from build123d import *

# Parameters (mm, degrees)
SKETCH_1_R      = 15
SKETCH_1_R_2    = 2.1
EXTRUDE_1_DEPTH = 7
EXTRUDE_START   = -2
SKETCH_2_R      = 17.5
SKETCH_2_R_2    = 2.1
EXTRUDE_2_DEPTH = 2
SKETCH_5_R      = 17.5
SKETCH_5_R_2    = 2.1
EXTRUDE_4_DEPTH = 1


with BuildPart() as part:
    # 草图1 → 凸台-拉伸1 (new body)
    with BuildSketch(Plane.XY):
        Circle(SKETCH_1_R)
        with Locations((0, 12)):
            Circle(SKETCH_1_R_2, mode=Mode.SUBTRACT)
        with Locations((10.392304845, 6)):
            Circle(SKETCH_1_R_2, mode=Mode.SUBTRACT)
        with Locations((10.392304845, -6)):
            Circle(SKETCH_1_R_2, mode=Mode.SUBTRACT)
        with Locations((0, -12)):
            Circle(SKETCH_1_R_2, mode=Mode.SUBTRACT)
        with Locations((-10.392304845, -6)):
            Circle(SKETCH_1_R_2, mode=Mode.SUBTRACT)
        with Locations((-10.392304845, 6)):
            Circle(SKETCH_1_R_2, mode=Mode.SUBTRACT)
        with Locations((4.425, 7.664324823)):
            Circle(SKETCH_1_R_2, mode=Mode.SUBTRACT)
        with Locations((4.419693866, -7.655134331)):
            Circle(SKETCH_1_R_2, mode=Mode.SUBTRACT)
        with Locations((-8.844693866, 0.009190493)):
            Circle(SKETCH_1_R_2, mode=Mode.SUBTRACT)
    extrude(amount=EXTRUDE_1_DEPTH)

    # 草图2 → 凸台-拉伸2 (add)
    with BuildSketch(Plane.XY.offset(7).offset(EXTRUDE_START)):
        Circle(SKETCH_2_R)
        with Locations((-8.844693866, 0.009190493)):
            Circle(SKETCH_2_R_2, mode=Mode.SUBTRACT)
        with Locations((-10.392304845, -6)):
            Circle(SKETCH_2_R_2, mode=Mode.SUBTRACT)
        with Locations((0, -12)):
            Circle(SKETCH_2_R_2, mode=Mode.SUBTRACT)
        with Locations((4.419693866, -7.655134331)):
            Circle(SKETCH_2_R_2, mode=Mode.SUBTRACT)
        with Locations((10.392304845, -6)):
            Circle(SKETCH_2_R_2, mode=Mode.SUBTRACT)
        with Locations((10.392304845, 6)):
            Circle(SKETCH_2_R_2, mode=Mode.SUBTRACT)
        with Locations((4.425, 7.664324823)):
            Circle(SKETCH_2_R_2, mode=Mode.SUBTRACT)
        with Locations((0, 12)):
            Circle(SKETCH_2_R_2, mode=Mode.SUBTRACT)
        with Locations((-10.392304845, 6)):
            Circle(SKETCH_2_R_2, mode=Mode.SUBTRACT)
    extrude(amount=EXTRUDE_2_DEPTH)

    # 草图5 → 凸台-拉伸4 (add)
    with BuildSketch(Plane.XY.offset(7)):
        Circle(SKETCH_5_R)
        with Locations((-10.392304845, -6)):
            Circle(SKETCH_5_R_2, mode=Mode.SUBTRACT)
        with Locations((0, -12)):
            Circle(SKETCH_5_R_2, mode=Mode.SUBTRACT)
        with Locations((4.419693866, -7.655134331)):
            Circle(SKETCH_5_R_2, mode=Mode.SUBTRACT)
        with Locations((10.392304845, -6)):
            Circle(SKETCH_5_R_2, mode=Mode.SUBTRACT)
        with Locations((10.392304845, 6)):
            Circle(SKETCH_5_R_2, mode=Mode.SUBTRACT)
        with Locations((4.425, 7.664324823)):
            Circle(SKETCH_5_R_2, mode=Mode.SUBTRACT)
        with Locations((0, 12)):
            Circle(SKETCH_5_R_2, mode=Mode.SUBTRACT)
        with Locations((-8.844693866, 0.009190493)):
            Circle(SKETCH_5_R_2, mode=Mode.SUBTRACT)
        with Locations((-10.392304845, 6)):
            Circle(SKETCH_5_R_2, mode=Mode.SUBTRACT)
    extrude(amount=EXTRUDE_4_DEPTH)


solid = part.part
Design review of the part built by this model. Coordinates are the model's own, in mm. A direction names the side the tool comes from. Round coordinates to 2 decimals unless told otherwise and drop trailing zeros. Loops run counter-clockwise (first coordinate to the right, second up) from the corner with the lowest first, then second, coordinate; pieces in that order, holes last. Notation, with made-up numbers: M 52,-20.5 L 80,-20.5 A31 ccw 80,8.5 Z; hole C 73,-36 d5. An arc over 180 degrees is marked long. Answer as a JSON object with one key per item and string values.
Item 1: Machinability: for faces 4 (the flat face through (13, 8, 5)), 5 (the cylindrical face through (8.845, 7.419, 3.944)), which of the approach directions +Z, -Z, +X, -X, +Y, -Y give a long, thin tool a straight path to every point of the face, cutting with its end or side? Answer none if there is none.
Answer sheet:
{"face 4": "-Z", "face 5": "+Z, -Z"}
Item 2: Wall thickness on L1, parallel to Y at x = 0, z = 1.5; L2, parallel to Y at x = 0, z = 6.25; L3, parallel to X at y = -7.5, z = 2: over which ranges is each line inside the solid? List them lowest first. Write a range as from..to.
Answer sheet:
{"L1": "y = -15..-14.1, -9.9..9.9, 14.1..15", "L2": "y = -17.5..-14.1, -9.9..9.9, 14.1..17.5", "L3": "x = -12.99..-11.86, -8.92..2.33, 6.51..8.92, 11.86..12.99"}
Item 3: Clearance check with flat-ended pins moving along their axes: P1, Ø4, axis at x = 0, y = 12, coming from the -Z side; P2, Ø3, axis at y = 12.5, z = 7, coming from the +X side; P3, Ø4, axis at x = 11.5, z = 6.5, coming from the +Y side; P4, Ø3, axis at y = -7, z = 3, coming from the -X side. State where each tip first meets the part, or that it passes through.
Answer sheet:
{"P1": "passes through", "P2": "stops at x = 13.61", "P3": "stops at y = 14.7", "P4": "stops at x = -13.96"}
Item 4: We need section D-D on y = 10.5. Give the boundary of the cut face in (x, z), and give its area (3 significant figures).
Answer sheet:
{"outline": "M -14,5 L -10.71,5 L -10.71,0 L -1.47,0 L -1.47,8 L -14,8 Z; M 1.47,0 L 10.71,0 L 10.71,5 L 14,5 L 14,8 L 1.47,8 Z", "area": "168 mm^2"}
Item 5: We need section C-C on y = 6. Give the boundary of the cut face in (x, z), and give its area (3 significant figures).
Answer sheet:
{"outline": "M -16.44,5 L -13.75,5 L -13.75,0 L -12.49,0 L -12.49,8 L -16.44,8 Z; M -8.29,0 L 3.14,0 L 3.14,8 L -8.29,8 Z; M 5.71,0 L 8.29,0 L 8.29,8 L 5.71,8 Z; M 12.49,0 L 13.75,0 L 13.75,5 L 16.44,5 L 16.44,8 L 12.49,8 Z", "area": "148 mm^2"}
Item 6: We need section B-B on y = -12. Give the boundary of the cut face in (x, z).
Answer sheet:
{"outline": "M -12.74,5 L -9,5 L -9,0 L -2.1,0 L -2.1,8 L -12.74,8 Z; M 2.1,0 L 9,0 L 9,5 L 12.74,5 L 12.74,8 L 2.1,8 Z"}
Item 7: The part is to be moulded in two halves that separate along X. For faces 1 (the flat face through (0, 0, 0)), 2 (the cylindrical face through (8.73, -7.28, 3.94)), 3 (the cylindrical face through (-13.887, -10.648, 6.479)), say which applies: pulls with the +X half, pulls with the -X half, needs draft (parallel to the pull), parting line crosses it, or undercut.
Answer sheet:
{"face 1": "needs draft", "face 2": "undercut", "face 3": "parting line crosses it"}
Item 8: We need section A-A on x = 0. Give the boundary of the cut face in (y, z).
Answer sheet:
{"outline": "M -17.5,5 L -15,5 L -15,0 L -14.1,0 L -14.1,8 L -17.5,8 Z; M -9.9,0 L 9.9,0 L 9.9,8 L -9.9,8 Z; M 14.1,0 L 15,0 L 15,5 L 17.5,5 L 17.5,8 L 14.1,8 Z"}
